Could you check a few things on this model? Use its own coordinates, in mm. A direction names the side the tool comes from. Coordinates: 2 decimals unless noted, no trailing zeros. Order: outer loops, then holes, each group sorted by start corner. A loop starts at its lowest first (then second) coordinate and runs counter-clockwise, first axis right, second up. Notation, with made-up numbers: (-32.5, -19.5) - (16.5, -19.5) arc R8 cw to (16.5, -10.5) - close; hole circle Ø10 at (48.25, -28). An arc over 180 degrees is marked (long way). Answer as a JSON object with one key per item and string values. Group by question number.
(1) Imagine slicing it at D-D, the plane z = 9.75. Write out the boundary of the cut face in (x, y), and give its area (3 significant figures).
(2) Imagine slicing it at C-C, the plane y = 1.5. Write out the boundary of the cut face in (x, z), and give its area (3 significant figures).
(3) We'd pull the mould along X, two halves only. Please class faces 3 (the flat face through (0, 12, 6)), 4 (the cylindrical face through (5.324, 2.354, 3.698)), 5 (the flat face through (10, 24.5, 6)), 6 (the cylindrical face through (9.905, 5.367, 9.472)): pulls with the +X half, pulls with the -X half, needs draft (parallel to the pull), parting line crosses it, or undercut.
(4) Which directions (+Z, -Z, +X, -X, +Y, -Y) give clear straight access to the entire face, cutting with the end or side of a thin tool? Please do faces 1 (the cylindrical face through (6, 17, 9)), 2 (the cylindrical face through (5.324, 18.854, 3.698)).
(5) Will this pin go through, and if not, where does the flat tip stop? P1, Ø2, axis at x = 6.5, y = 22.5, coming from the +Z side.
(6) Please list where these lines run through material, in increasing order: probe 1 along X at (y, z) = (4.5, 10.6); probe 2 along Y at (x, z) = (6, 9.85); probe 3 along Y at (x, z) = (17.25, 2.5).
(7) Imagine slicing it at B-B, the plane x = 6. Write out the boundary of the cut face in (y, z).
(8) Imagine slicing it at A-A, the plane y = 21. Write out the boundary of the cut face in (x, z).
Autodesk Inventor part; units mm, degrees
ref_plane "YZ Plane" through (0, 0, 0) normal (1, 0, 0) x (0, 1, 0)
ref_plane "XZ Plane" through (0, 0, 0) normal (0, 1, 0) x (-1, 0, 0)
ref_plane "XY Plane" through (0, 0, 0) normal (0, 0, 1) x (1, 0, 0)
sketch "Sketch1" plane through (0, 0, 0) normal (0, 0, 1) x (1, 0, 0)
  line L0 (0, 0) -> (19.5, 0)
  line L1 (19.5, 0) -> (19.5, 24.5)
  line L2 (19.5, 24.5) -> (0, 24.5)
  line L3 (0, 24.5) -> (0, 0)
  dimension "d0" = 24.5
  dimension "d1" = 19.5
extrude "Extrusion1" add sketch "Sketch1" along normal blind 11.5
sketch "Sketch2" plane through (0, 0, 11.5) normal (0, 0, 1) x (1, 0, 0)
  line L0 (0, 0) -> (19.5, 0)
  line L1 (0, 24.5) -> (0, 0)
  point P0 (6, 21)
  point P1 (6, 4.5)
  dimension "d4" = 4.5
  dimension "d5" = 6
  dimension "d27" = 16.5
hole "Hole1" at (6, 21, 11.5) at (6, 4.5, 11.5) direction (0, 0, -1) diameter 4.5 end up to surface counterbore diameter 8 counterbore depth 4
sketch "Sketch4" plane through (0, 0, 0) normal (-1, 0, 0) x (0, 0, 1)
  line L0 (0, 24.5) -> (0, 0)
  line L1 (0, 24.5) -> (11.5, 24.5)
  circle A0 centre (-0.5, 14.5) radius 4.1
  dimension "d19" = 8.2
  dimension "d20" = 0.5
  dimension "d21" = 10
extrude "Extrusion3" cut sketch "Sketch4" against normal up to surface (19.5 mm away)
sketch "Sketch5" plane through (6, 21, 7.5) normal (0, 0, 1) x (1, 0, 0)
  circle A0 centre (0, 0) radius 4
  circle A1 centre (0, -16.5) radius 3.5
  circle A2 centre (0, -16.5) radius 2
  point P0 (-6, -21)
properties part number "YIdlerCapLeft" material "ABS Plastic"
Result set:
{
 "1": {"outline": "(0, 0) - (19.5, 0) - (19.5, 24.5) - (7.94, 24.5) arc R4 cw (long way) to (4.06, 24.5) - (0, 24.5) - close; hole circle Ø8 at (6, 4.5)", "area": "379 mm^2"},
 "2": {"outline": "(0, 0) - (19.5, 0) - (19.5, 11.5) - (8.65, 11.5) - (8.65, 7.5) - (3.35, 7.5) - (3.35, 11.5) - (0, 11.5) - close", "area": "203 mm^2"},
 "3": {"face 3": "pulls with the -X half", "face 4": "undercut", "face 5": "needs draft", "face 6": "undercut"},
 "4": {"face 1": "+Z", "face 2": "+Z, -Z"},
 "5": {"P1": "stops at z = 7.5"},
 "6": {"probe 1": "x = 0 to 2, 10 to 19.5", "probe 2": "y = 0 to 0.5, 8.5 to 17", "probe 3": "y = 0 to 11.71, 17.29 to 24.5"},
 "7": {"outline": "(0, 0) - (2.25, 0) - (2.25, 7.5) - (0.5, 7.5) - (0.5, 11.5) - (0, 11.5) - close; (6.75, 0) - (10.43, 0) arc R4.1 cw to (18.57, 0) - (18.75, 0) - (18.75, 7.5) - (17, 7.5) - (17, 11.5) - (8.5, 11.5) - (8.5, 7.5) - (6.75, 7.5) - close; (23.25, 0) - (24.5, 0) - (24.5, 7.5) - (23.25, 7.5) - close"},
 "8": {"outline": "(0, 0) - (3.75, 0) - (3.75, 7.5) - (2, 7.5) - (2, 11.5) - (0, 11.5) - close; (8.25, 0) - (19.5, 0) - (19.5, 11.5) - (10, 11.5) - (10, 7.5) - (8.25, 7.5) - close"}
}
